from build123d import *

# Parameters (mm, degrees)
SKETCH_1_R          = 1.5
EXTRUDE_1_DEPTH     = 3
SKETCH_2_R          = 8.856274186
SKETCH_2_R_2        = 1.600284684
SKETCH_2_R_3        = 1.750181187
SKETCH_2_R_4        = 1.993052337
SKETCH_2_W          = 53.334767433
SKETCH_2_H          = 4.299974178
CUT_EXTRUDE_1_DEPTH = 42.716303767


with BuildPart() as part:
    # 草图1 → 凸台-拉伸1 (new body)
    with BuildSketch(Plane(origin=(0, 0, 0), x_dir=(1, 0, 0), z_dir=(0, 1, 0))):
        with BuildLine():
            Line((-30, 22.5), (30, 22.5))
            ThreePointArc((30, 22.5), (33.535533906, 21.035533906), (35, 17.5))
            Line((35, 17.5), (35, -17.5))
            ThreePointArc((35, -17.5), (33.535533906, -21.035533906), (30, -22.5))
            Line((30, -22.5), (-30, -22.5))
            ThreePointArc((-30, -22.5), (-33.535533906, -21.035533906), (-35, -17.5))
            Line((-35, -17.5), (-35, 17.5))
            ThreePointArc((-35, 17.5), (-33.535533906, 21.035533906), (-30, 22.5))
        make_face()
        with Locations(Location((-30.4, -17.95, 0), (0, 0, 270))):
            Circle(SKETCH_1_R, mode=Mode.SUBTRACT)
        with Locations(Location((30.4, -17.95, 0), (0, 0, 90))):
            Circle(SKETCH_1_R, mode=Mode.SUBTRACT)
        with Locations(Location((30.4, 17.95, 0), (0, 0, 270))):
            Circle(SKETCH_1_R, mode=Mode.SUBTRACT)
        with Locations(Location((-30.4, 17.95, 0), (0, 0, 90))):
            Circle(SKETCH_1_R, mode=Mode.SUBTRACT)
    extrude(amount=EXTRUDE_1_DEPTH)

    # 草图2 → 切除-拉伸1 (cut, through all)
    with BuildSketch(Plane(origin=(0, 3, 0), x_dir=(1, 0, 0), z_dir=(0, 1, 0))):
        with Locations(Location((0, 0, 0), (0, 0, 270))):
            Circle(SKETCH_2_R)
        with Locations(Location((-31.892993618, 12.805189582, 0), (0, 0, 270))):
            Circle(SKETCH_2_R_2)
        with Locations(Location((-31.892993618, 0, 0), (0, 0, 270))):
            Circle(SKETCH_2_R_3)
        with Locations(Location((-31.892993618, -13.094810418, 0), (0, 0, 270))):
            Circle(SKETCH_2_R_4)
        with Locations((0.339471646, -18.029716289)):
            Rectangle(SKETCH_2_W, SKETCH_2_H)
    extrude(amount=-CUT_EXTRUDE_1_DEPTH, mode=Mode.SUBTRACT)


solid = part.part
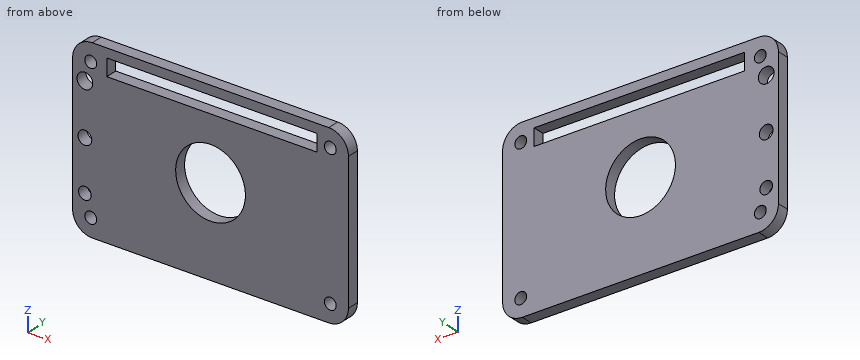
Verification items for the finished model (mm, model axes). Give positions to 0.01 mm unless a question says otherwise; leave off trailing zeros. Write each loop counter-clockwise with the first axis right and the second up, starting at its lowest first coordinate (ties: lowest second). Pieces come first, ordered by that corner, then holes. Notation, with made-up numbers: M 15,-11 L 60,-11 A22 ccw 60,24 Z; hole C -19,-9.5 d6. An arc over 180 degrees is marked long. Use CSV: the item, a comma, the result in double quotes.
1) Material ranges on line 1 along X through (y, z) = (1.3, 0); line 2 along Z through (x, y) = (-1, 2.8); line 3 along Z through (x, y) = (-16, 0.55), recorded low to high.
Final values:
line 1,"-35 to -33.64, -30.14 to -8.86, 8.86 to 35"
line 2,"-22.5 to -8.8, 8.8 to 15.88, 20.18 to 22.5"
line 3,"-22.5 to 15.88, 20.18 to 22.5"
2) Cross-section at A-A (x = 0). Enter the section's corners in (y, z), plus the area to 3 significant figures.
Final values:
outline,"M 0,-22.5 L 3,-22.5 L 3,-8.86 L 0,-8.86 Z; M 0,8.86 L 3,8.86 L 3,15.88 L 0,15.88 Z; M 0,20.18 L 3,20.18 L 3,22.5 L 0,22.5 Z"
area,"69.0 mm²"
3) Cross-section at D-D (z = 14). Enter the section's corners in (x, y), plus the area to 3 significant figures.
Final values:
outline,"M -35,0 L -33.67,0 L -33.67,3 L -35,3 Z; M -30.12,0 L 35,0 L 35,3 L -30.12,3 Z"
area,"199 mm²"
4) Cross-section at B-B (x = -25). Enter the section's corners in (y, z).
Final values:
outline,"M 0,-22.5 L 3,-22.5 L 3,15.88 L 0,15.88 Z; M 0,20.18 L 3,20.18 L 3,22.5 L 0,22.5 Z"
5) Cross-section at C-C (z = 0). Enter the section's corners in (x, y).
Final values:
outline,"M -35,0 L -33.64,0 L -33.64,3 L -35,3 Z; M -30.14,0 L -8.86,0 L -8.86,3 L -30.14,3 Z; M 8.86,0 L 35,0 L 35,3 L 8.86,3 Z"
